```python
from build123d import *

# Parameters (mm, degrees)
BOSS_EXTRUDE1_DEPTH = 40
CHAMFER1_SIZE       = 28


with BuildPart() as part:
    # Sketch1 → Boss-Extrude1 (new body)
    with BuildSketch(Plane(origin=(0, 0, 0), x_dir=(1, 0, 0), z_dir=(0, 1, 0))):
        with BuildLine():
            Line((0, 0), (0, 17.5))
            Line((0, 17.5), (40, 17.5))
            Line((40, 17.5), (52.5, 30))
            Line((52.5, 30), (245, 30))
            Line((245, 30), (245, 11))
            Line((245, 11), (75, 11))
            ThreePointArc((75, 11), (64, 0), (75, -11))
            Line((75, -11), (245, -11))
            Line((245, -11), (245, -30))
            Line((245, -30), (52.5, -30))
            Line((52.5, -30), (40, -17.5))
            Line((40, -17.5), (0, -17.5))
            Line((0, -17.5), (0, 0))
        make_face()
    extrude(amount=BOSS_EXTRUDE1_DEPTH)

    # Chamfer1
    chamfer1_edges = [part.edges().sort_by_distance(p)[0] for p in [
        (0, 40, 0),
    ]]
    chamfer(chamfer1_edges, length=CHAMFER1_SIZE)


solid = part.part
```
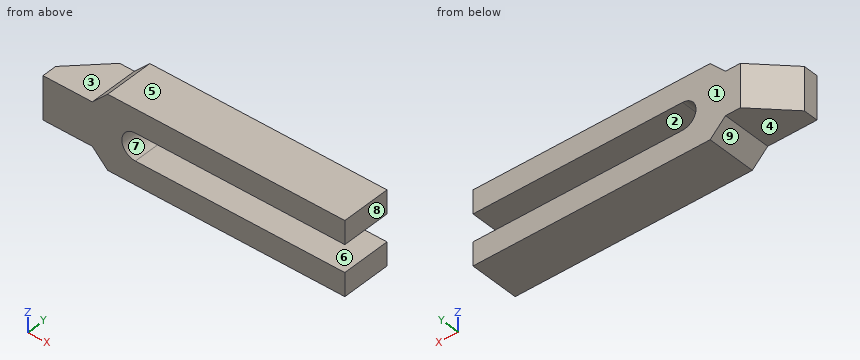
Geometry: final body of the model. Coordinates: model frame, mm. Face numbers are marked on the shaded views. A direction names the side the tool comes from. Round coordinates to 2 decimals unless told otherwise and drop trailing zeros. Write each loop counter-clockwise with the first axis right and the second up, starting at its lowest first coordinate (ties: lowest second). Pieces come first, ordered by that corner, then holes. Notation, with made-up numbers: M -19.5,-9 L 22.5,-9 A18 cw 22.5,12 Z; hole C -25,15.5 d1. An arc over 180 degrees is marked long. Answer in a Markdown table with one row per item. Add a question column.
(1) Contact query for flat-ended pins moving along their axis: pin 1 (12 mm diameter, centred on y = 21, z = 11.5, fed in from -X); pin 2 (12 mm diameter, centred on x = 27.5, y = 14.5, fed in from -Z); pin 3 (4 mm diameter, centred on x = 29, z = -16, fed in from -Y); pin 4 (12 mm diameter, centred on x = 10.5, y = 23.5, fed in from +Z). Output: stop coordinate, or through.
(2) Draft query along Z for the marked faces 6, 7, 8 and 9. Return one class per face: pulls with the +Z half, pulls with the -Z half, needs draft (parallel to the pull), parting line crosses it, or undercut.
(3) Cut plane B-B, the plane z = 0. Return the cut outline in (x, y).
(4) Ray query, L1, parallel to Z at x = 215, y = 32; L2, parallel to Z at x = 38, y = 36; L3, parallel to X at y = 4.5, z = -3.5. Return the intervals inside material, ascending.
(5) Cut plane C-C, the plane y = 29. Return the cut outline in (x, z), then the cut area to 3 significant figures.
(6) Cut plane A-A, the plane x = 219. Return the cut outline in (y, z), then the cut area to 3 significant figures.
(7) Reachability of the marked faces 1, 2, 3, 4 and 5 from +Z, -Z, +X, -X, +Y, -Y: full face, straight path, thin tool, end or side. Return the list, or none.
Established:
| question | item | result |
|---|---|---|
| 1 | pin 1 | x = 3 |
| 1 | pin 2 | z = -17.5 |
| 1 | pin 3 | y = 0 |
| 1 | pin 4 | z = 17.5 |
| 2 | face 6 | undercut |
| 2 | face 7 | undercut |
| 2 | face 8 | needs draft |
| 2 | face 9 | pulls with the -Z half |
| 3 | outline | M 0,0 L 64,0 L 64,40 L 28,40 L 0,12 Z |
| 4 | L1 | -30 to -11, 11 to 30 |
| 4 | L2 | -17.5 to 17.5 |
| 4 | L3 | 0 to 64.57 |
| 5 | outline | M 17,-17.5 L 40,-17.5 L 52.5,-30 L 245,-30 L 245,-11 L 75,-11 A11 cw 75,11 L 245,11 L 245,30 L 52.5,30 L 40,17.5 L 17,17.5 Z |
| 5 | area | 9,020 mm² |
| 6 | outline | M 0,-30 L 40,-30 L 40,-11 L 0,-11 Z; M 0,11 L 40,11 L 40,30 L 0,30 Z |
| 6 | area | 1,520 mm² |
| 7 | face 1 | +Z, -Z, +X, -X, +Y |
| 7 | face 2 | +X, +Y, -Y |
| 7 | face 3 | +Z, -X, +Y, -Y |
| 7 | face 4 | -Z, -X, +Y, -Y |
| 7 | face 5 | +Z, +X, -X, +Y, -Y |
